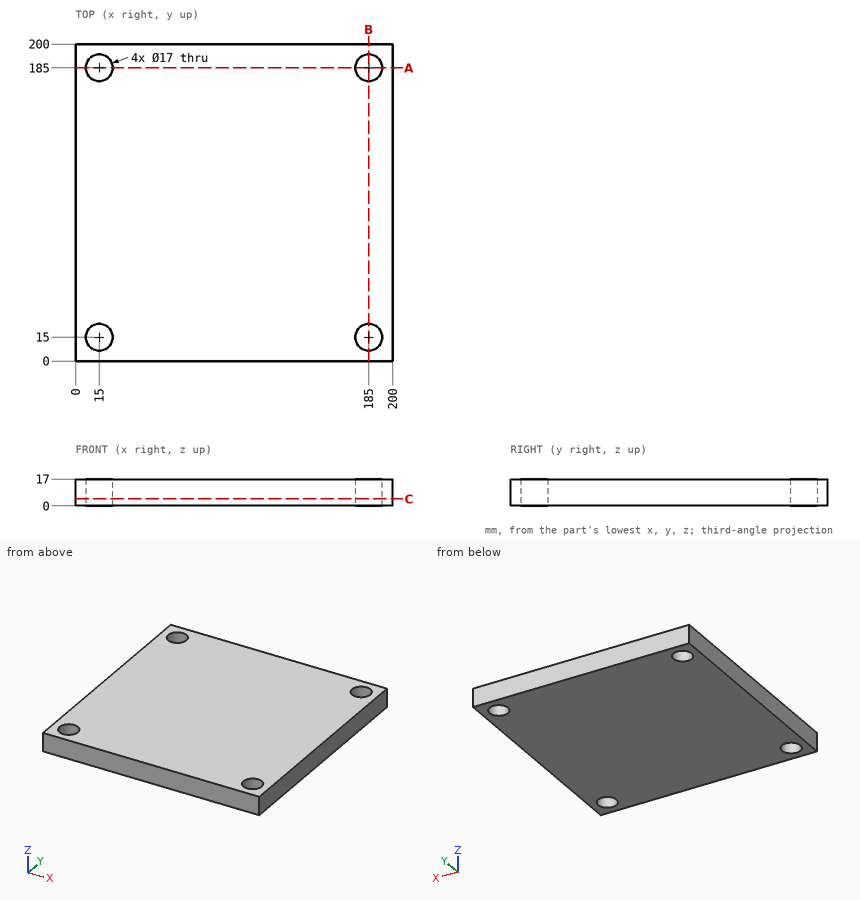
Answer from the drawing. Dimensions are ordinates in mm from the lowest x, y and z of the part. Give positions to 0.01 mm unless a question says otherwise; leave off trailing zeros. Write each loop counter-clockwise with the first axis right and the second up, starting at its lowest first coordinate (ties: lowest second). Pieces come first, ordered by that corner, then holes. Notation, with made-up numbers: (88, 31.25) -> (145, 31.25) arc R27 cw to (145, 62.25) -> close; hole circle Ø6 at (-25.75, 29). An arc over 180 degrees is marked (long way). Use a Markdown table: item, result.
(1) A flat-ended cylindrical pin translates along its axis: P1, Ø13.5, axis at x = 185, y = 185, coming from the -Z side. Find the tip coordinate at first contact, or state that the pin passes through.
Return value:
| item | result |
|---|---|
| P1 | through |
(2) Section A-A, the plane y = 185 is taken. Determine the outline of the cut face in (x, z), then the cut area to 3 significant figures.
Return value:
| item | result |
|---|---|
| outline | (0, 0) -> (6.5, 0) -> (6.5, 17) -> (0, 17) -> close; (23.5, 0) -> (176.5, 0) -> (176.5, 17) -> (23.5, 17) -> close; (193.5, 0) -> (200, 0) -> (200, 17) -> (193.5, 17) -> close |
| area | 2,820 mm2 |
(3) Find the intervals of material crossed by probe 1 along X at (y, z) = (15, 5.5); probe 2 along Y at (x, z) = (186.5, 2.25), in increasing order. Write a range as from..to.
Return value:
| item | result |
|---|---|
| probe 1 | 0..6.5, 23.5..176.5, 193.5..200 |
| probe 2 | 0..6.63, 23.37..176.63, 193.37..200 |
(4) Section C-C, the plane z = 4.5 is taken. Determine the outline of the cut face in (x, y), then the cut area to 3 significant figures.
Return value:
| item | result |
|---|---|
| outline | (0, 0) -> (200, 0) -> (200, 200) -> (0, 200) -> close; hole circle Ø17 at (15, 15); hole circle Ø17 at (15, 185); hole circle Ø17 at (185, 15); hole circle Ø17 at (185, 185) |
| area | 39,100 mm2 |
